from build123d import *

# Parameters (mm, degrees)
SKETCH_1_W               = 100
SKETCH_1_H               = 100
EXTRUDE_1_DEPTH          = 18
SKETCH_2_W               = 50
SKETCH_2_H               = 30
CUT_EXTRUDE_1_DEPTH      = 13
CUT_EXTRUDE_2_DEPTH      = 72.895757872
CUT_EXTRUDE_2_DEPTH_BACK = 72.895757872
SKETCH_4_W               = 33
SKETCH_4_H               = 28.5
CUT_EXTRUDE_3_DEPTH      = 9


with BuildPart() as part:
    # Эскиз1 → Бобышка-Вытянуть1 (new body)
    with BuildSketch(Plane(origin=(0, 0, 0), x_dir=(1, 0, 0), z_dir=(0, 1, 0))):
        Rectangle(SKETCH_1_W, SKETCH_1_H)
    extrude(amount=EXTRUDE_1_DEPTH)

    # Эскиз2 → Вырез-Вытянуть1 (cut)
    with BuildSketch(Plane(origin=(0, 18, 0), x_dir=(1, 0, 0), z_dir=(0, 1, 0))):
        with Locations((0, -20.616579454)):
            Rectangle(SKETCH_2_W, SKETCH_2_H)
    extrude(amount=-CUT_EXTRUDE_1_DEPTH, mode=Mode.SUBTRACT)

    # Эскиз3 → Вырез-Вытянуть2 (cut, two sides: drawn at the far end of the back side and taken through both)
    with BuildSketch(Plane(origin=(0, 5, 0), x_dir=(1, 0, 0), z_dir=(0, 1, 0)).offset(-CUT_EXTRUDE_2_DEPTH_BACK)):
        with BuildLine():
            Line((10, -31.116579454), (-10, -31.116579454))
            ThreePointArc((-10, -31.116579454), (-13.535533906, -29.65211336), (-15, -26.116579454))
            Line((-15, -26.116579454), (-15, -12.616579454))
            ThreePointArc((-15, -12.616579454), (-13.535533906, -9.081045548), (-10, -7.616579454))
            Line((-10, -7.616579454), (10, -7.616579454))
            ThreePointArc((10, -7.616579454), (13.535533906, -9.081045548), (15, -12.616579454))
            Line((15, -12.616579454), (15, -26.116579454))
            ThreePointArc((15, -26.116579454), (13.535533906, -29.65211336), (10, -31.116579454))
        make_face()
    extrude(amount=CUT_EXTRUDE_2_DEPTH + CUT_EXTRUDE_2_DEPTH_BACK, mode=Mode.SUBTRACT)

    # Эскиз4 → Вырез-Вытянуть3 (cut)
    with BuildSketch(Plane(origin=(0, 18, 0), x_dir=(1, 0, 0), z_dir=(0, 1, 0))):
        with Locations((0, 8.633420546)):
            Rectangle(SKETCH_4_W, SKETCH_4_H)
    extrude(amount=-CUT_EXTRUDE_3_DEPTH, mode=Mode.SUBTRACT)


solid = part.part
Work out the finished part from the listing and answer in its coordinate system (mm). A direction names the side the tool comes from. Give positions to 0.01 mm unless a question says otherwise; leave off trailing zeros. Order: outer loops, then holes, each group sorted by start corner. A loop starts at its lowest first (then second) coordinate and runs counter-clockwise, first axis right, second up. Notation, with made-up numbers: (76.5, 84) -> (111.5, 84) arc R31 ccw to (111.5, 109) -> close; hole circle Ø2 at (72, 51.25). An arc over 180 degrees is marked (long way). One line per item, written item: value.
Item 1: Flat-ended cylindrical pins translate along their axes: P1, Ø4, axis at x = -27.5, z = -5.5, coming from the -Y side; P2, Ø14, axis at x = -0.5, z = -4, coming from the +Y side. Find the tip coordinate at first contact, or state that the pin passes through.
Answer sheet:
P1: y = 0
P2: y = 9
Item 2: Straight lines are drawn through the part: probe 1 along Z at (x, y) = (-12, 14.25); probe 2 along X at (y, z) = (12.5, -11); probe 3 along X at (y, z) = (15, 23.5). For each, find the intervals that lie inside material, in ascending order.
Answer sheet:
probe 1: -50 to -22.88, 35.62 to 50
probe 2: -50 to -16.5, 16.5 to 50
probe 3: -50 to -25, 25 to 50
Item 3: Find section B-B, the plane y = 10.75. Give the vertices of the cut face in (x, z).
Answer sheet:
outline: (-50, -50) -> (50, -50) -> (50, 50) -> (-50, 50) -> close; hole (-25, 5.62) -> (-16.5, 5.62) -> (-16.5, -22.88) -> (16.5, -22.88) -> (16.5, 5.62) -> (25, 5.62) -> (25, 35.62) -> (-25, 35.62) -> close
Item 4: Determine the mould class of faces 1 (the flat face through (-23, 18, -1)), 2 (the flat face through (0, 12, 35.617)), 3 (the cylindrical face through (13.574, 2.465, 29.613)), 4 (the flat face through (-50, 9, 1)) for opening direction X: released by +X, released by -X, zero draft, split by the parting line, or undercut.
Answer sheet:
face 1: zero draft
face 2: undercut
face 3: undercut
face 4: released by -X
Item 5: Find section C-C, the plane z = 22.5. Give the vertices of the cut face in (x, y).
Answer sheet:
outline: (-50, 0) -> (-15, 0) -> (-15, 5) -> (-25, 5) -> (-25, 18) -> (-50, 18) -> close; (15, 0) -> (50, 0) -> (50, 18) -> (25, 18) -> (25, 5) -> (15, 5) -> close
Item 6: Find section A-A, the plane x = 6. Give the vertices of the cut face in (y, z).
Answer sheet:
outline: (0, -50) -> (18, -50) -> (18, -22.88) -> (9, -22.88) -> (9, 5.62) -> (5, 5.62) -> (5, 7.62) -> (0, 7.62) -> close; (0, 31.12) -> (5, 31.12) -> (5, 35.62) -> (18, 35.62) -> (18, 50) -> (0, 50) -> close
Item 7: Find section D-D, the plane x = 18. Give the vertices of the cut face in (y, z).
Answer sheet:
outline: (0, -50) -> (18, -50) -> (18, 5.62) -> (5, 5.62) -> (5, 35.62) -> (18, 35.62) -> (18, 50) -> (0, 50) -> close
Item 8: A tool of negligible diameter and unlimited length cuts with its end or side. For faces 5 (the flat face through (-15, 2, 19)), 6 (the flat face through (25, 12, 21)), 7 (the flat face through (50, 9, 1)), from which of +Z, -Z, +X, -X, +Y, -Y can it reach the whole face along a straight path? Write none if from no direction.
Answer sheet:
face 5: +Y, -Y
face 6: +Y
face 7: +Z, -Z, +X, +Y, -Y
